```python
from build123d import *

# Parameters (mm, degrees)
F0_W      = 76.2
F0_H      = 88.9
F1_DEPTH  = 6.35
F2_W      = 6.6139022768
F2_H      = 88.9
F3_DEPTH  = 16.51
F4_W      = 69.5860977232
F4_H      = 6.2766113102
F5_DEPTH  = 12.7
F6_W      = 7.1120927989
F6_H      = 82.6233886898
F7_DEPTH  = 12.7
F8_W      = 62.4740049243
F8_H      = 7.9619140148
F9_DEPTH  = 12.7
F10_W     = 9.7436904907
F10_H     = 6.4433701336
F11_DEPTH = 6.35
F12_R     = 4.9368995646
F13_DEPTH = 6.35


with BuildPart() as f1:
    # F0 (on Top) → F1 (new body)
    with BuildSketch(Plane.XY):
        Rectangle(F0_W, F0_H)
    extrude(amount=F1_DEPTH)

    # F2 (on face) → F3 (join)
    with BuildSketch(Plane.XY.offset(6.35)):
        with Locations((34.7930488616, 0)):
            Rectangle(F2_W, F2_H)
    extrude(amount=F3_DEPTH)

    # F4 (on face) → F5 (join)
    with BuildSketch(Plane.XY.offset(6.35)):
        with Locations((-3.3069511384, -41.3116943449)):
            Rectangle(F4_W, F4_H)
    extrude(amount=F5_DEPTH)

    # F6 (on face) → F7 (join)
    with BuildSketch(Plane.XY.offset(6.35)):
        with Locations((-34.5439536005, 3.1383056551)):
            Rectangle(F6_W, F6_H)
    extrude(amount=F7_DEPTH)

    # F8 (on face) → F9 (join)
    with BuildSketch(Plane.XY.offset(6.35)):
        with Locations((0.2490952611, 40.4690429926)):
            Rectangle(F8_W, F8_H)
    extrude(amount=F9_DEPTH)

    # F10 (on face) → F11 (join)
    with BuildSketch(Plane.YZ.offset(38.1)):
        with Locations((0, 13.9397662133)):
            Rectangle(F10_W, F10_H)
    extrude(amount=F11_DEPTH)

    # F12 (on face) → F13 (join)
    with BuildSketch(Plane.YZ.offset(44.45)):
        with Locations((0, 13.8416578993)):
            Circle(F12_R)
    extrude(amount=F13_DEPTH)


solid = f1.part
```
Could you check a few things on this model? Use its own coordinates, in mm. A direction names the side the tool comes from. Give positions to 0.01 mm unless a question says otherwise; leave off trailing zeros. Order: outer loops, then holes, each group sorted by start corner. A loop starts at its lowest first (then second) coordinate and runs counter-clockwise, first axis right, second up.
Q1. Suppose I cut it at D-D, the plane y = 0. Write out the boundary of the cut face in (x, z), and give its area (3 significant figures).
Q2. Suppose I cut it at B-B, the plane x = 20.5. Write out the boundary of the cut face in (y, z), and give its area (3 significant figures).
Q3. Suppose I cut it at A-A, the plane y = 14. Write out the boundary of the cut face in (x, z), and give its area (3 significant figures).
Q4. We'd pull the mould along X, two halves only. Please class faces 1 (the flat face through (0, 0, 6.35)), 2 (the flat face through (-1, 44.45, 11)), 3 (the flat face through (41, 0, 10.718)), 4 (the flat face through (50.8, 0, 14)): +X half, -X half, draft (parallel to the pull), parting line (faces both ways), or undercut.
Q5. If I drill on line 1 along X through (y, z) = (2, 15.75); line 2 along X through (y, z) = (-26, 9.5); line 3 along Y through (x, z) = (0.5, 11.75), over which ranges is the centre line in solid material (lowest first)?
Q6. I'm going to push flat-ended pins straight in: P1, Ø1.9, axis at x = 41, z = 15, coming from the -Y side; P2, Ø1.5, axis at y = -21.5, z = 14.5, coming from the +X side; P3, Ø3, axis at x = 40, y = 2, coming from the -Z side. Where does each tip first touch, or does it pass through?
Q7. For faces 5 (the flat face through (41, 0, 17.161)), 6 (the cylindrical face through (47.581, -0.643, 18.737)), 7 (the flat face through (-32, 0, 19.05)), 8 (the flat face through (0, 36.488, 13)), which set-ups out of +Z, -Z, +X, -X, +Y, -Y let a thin tool reach every point of the face, with its end or its side?
Q8. Suppose I cut it at C-C, the plane z = 4. Write out the boundary of the cut face in (x, y), and give its area (3 significant figures).
Solution:
1. outline: (-38.1, 0) - (38.1, 0) - (38.1, 10.72) - (44.45, 10.72) - (44.45, 8.9) - (50.8, 8.9) - (50.8, 18.78) - (44.45, 18.78) - (44.45, 17.16) - (38.1, 17.16) - (38.1, 22.86) - (31.49, 22.86) - (31.49, 6.35) - (-30.99, 6.35) - (-30.99, 19.05) - (-38.1, 19.05) - close
1. area: 787 mm2
2. outline: (-44.45, 0) - (44.45, 0) - (44.45, 19.05) - (36.49, 19.05) - (36.49, 6.35) - (-38.17, 6.35) - (-38.17, 19.05) - (-44.45, 19.05) - close
2. area: 745 mm2
3. outline: (-38.1, 0) - (38.1, 0) - (38.1, 22.86) - (31.49, 22.86) - (31.49, 6.35) - (-30.99, 6.35) - (-30.99, 19.05) - (-38.1, 19.05) - close
3. area: 683 mm2
4. face 1: undercut
4. face 2: draft
4. face 3: undercut
4. face 4: +X half
5. line 1: x = -38.1 to -30.99, 31.49 to 50.8
5. line 2: x = -38.1 to -30.99, 31.49 to 38.1
5. line 3: y = -44.45 to -38.17, 36.49 to 44.45
6. P1: stops at y = -4.87
6. P2: stops at x = 38.1
6. P3: stops at z = 10.72
7. face 5: +Z, +Y, -Y
7. face 6: +X
7. face 7: +Z, -X, +Y, -Y
7. face 8: +Z
8. outline: (-38.1, -44.45) - (38.1, -44.45) - (38.1, 44.45) - (-38.1, 44.45) - close
8. area: 6,770 mm2
